Build history of the part. All positions in model axes, mm. A direction names the side the tool comes from. Coordinates: 2 decimals unless noted, no trailing zeros. Loops run counter-clockwise (first coordinate to the right, second up) from the corner with the lowest first, then second, coordinate; pieces in that order, holes last. Notation, with made-up numbers: (47.25, 69) - (56.25, 69) arc R20 ccw to (56.25, 96) - close; hole circle Ø1 at (60.25, 48). An arc over 180 degrees is marked (long way). One line per item, written item: value.
```python
from build123d import *

# Parameters (mm, degrees)
ESBO_O2_R                           = 12.5
RESSALTO_EXTRUS_O1_DEPTH            = 5.55
RESSALTO_EXTRUS_O3_DEPTH            = 3
ESBO_O5_W                           = 25
ESBO_O5_H                           = 7.051040728
RESSALTO_EXTRUS_O4_DEPTH            = 11.8
REBAIXO_PARA_SHCS_M2_51_D           = 2.9
REBAIXO_PARA_SHCS_M2_51_CBORE_D     = 5.5
REBAIXO_PARA_SHCS_M2_51_CBORE_DEPTH = 10
NERVURA1_REACH                      = 67.976
ESBO_O10_WALL_W                     = 145.845066172
ESBO_O10_WALL_H                     = 15
CORTE_EXTRUS_O1_REACH               = 68.009
ESBO_O11_W                          = 9
ESBO_O11_H                          = 8
ESBO_O12_R                          = 3.25
CORTE_EXTRUS_O2_DEPTH               = 67.475439137
ESBO_O13_R                          = 4
CORTE_EXTRUS_O3_DEPTH               = 7.55


with BuildPart() as part:
    # Esboço2 → Ressalto-extrusão1 (new body)
    with BuildSketch(Plane.XY):
        with Locations((-0.474928023, -0.063425095)):
            Circle(ESBO_O2_R)
    extrude(amount=-RESSALTO_EXTRUS_O1_DEPTH)

    # Esboço4 → Ressalto-extrusão3 (add)
    with BuildSketch(Plane(origin=(0, 0, -5.55), x_dir=(-1, 0, 0), z_dir=(0, 0, -1))):
        with BuildLine():
            Line((-12.025071977, -0.063425095), (-12.025071977, 64.120162595))
            Line((-12.025071977, 64.120162595), (12.974928023, 64.120162595))
            Line((12.974928023, 64.120162595), (12.974928023, -0.063425095))
            ThreePointArc((12.974928023, -0.063425095), (0.474928023, -12.563425095), (-12.025071977, -0.063425095))
        make_face()
    extrude(amount=RESSALTO_EXTRUS_O3_DEPTH)

    # Esboço5 → Ressalto-extrusão4 (add)
    with BuildSketch(Plane(origin=(0, 0, -8.55), x_dir=(-1, 0, 0), z_dir=(0, 0, -1))):
        with Locations((0.474928023, 60.594642231)):
            Rectangle(ESBO_O5_W, ESBO_O5_H)
    extrude(amount=-RESSALTO_EXTRUS_O4_DEPTH)

    # Rebaixo para SHCS M2.51 (through all)
    with Locations(Plane(origin=(0, 0, -8.55), x_dir=(-1, 0, 0), z_dir=(0, 0, -1))):
        with Locations((-8.49949915, 61.707782077), (8.5, 61.838275999)):
            CounterBoreHole(REBAIXO_PARA_SHCS_M2_51_D / 2, REBAIXO_PARA_SHCS_M2_51_CBORE_D / 2, REBAIXO_PARA_SHCS_M2_51_CBORE_DEPTH)

    # Esboço10 wall → Nervura1 (add, up to next)
    with BuildSketch(Plane(origin=(0, 53.069121867, -1.15), x_dir=(0, -0.672672793996, -0.739940073396), z_dir=(0, 0.739940073396, -0.672672793996)), mode=Mode.PRIVATE) as nervura1_sk1:
        Rectangle(ESBO_O10_WALL_W, ESBO_O10_WALL_H)
    nervura1_tool1 = extrude(nervura1_sk1.sketch, amount=NERVURA1_REACH, mode=Mode.PRIVATE) - part.part
    add(nervura1_tool1.solids().sort_by_distance((0, 53.069121867, -1.15))[0])

    # Esboço11 → Corte-extrusão1 (cut, up to next)
    with BuildSketch(Plane.XY.offset(-5.55), mode=Mode.PRIVATE) as corte_extrus_o1_sk1:
        with Locations((0, 53.069121867)):
            Rectangle(ESBO_O11_W, ESBO_O11_H)
    corte_extrus_o1_tool1 = extrude(corte_extrus_o1_sk1.sketch, amount=CORTE_EXTRUS_O1_REACH, mode=Mode.PRIVATE) & part.part
    add(corte_extrus_o1_tool1.solids().sort_by_distance((0, 53.069122, -5.55))[0], mode=Mode.SUBTRACT)

    # Esboço12 → Corte-extrusão2 (cut, through all)
    with BuildSketch(Plane(origin=(0, 0, -8.55), x_dir=(-1, 0, 0), z_dir=(0, 0, -1))):
        with Locations((0.474928023, -0.063425095)):
            Circle(ESBO_O12_R)
    extrude(amount=-CORTE_EXTRUS_O2_DEPTH, mode=Mode.SUBTRACT)

    # Esboço13 → Corte-extrusão3 (cut)
    with BuildSketch(Plane(origin=(0, 0, -8.55), x_dir=(-1, 0, 0), z_dir=(0, 0, -1))):
        with Locations((0.474928023, -0.063425095)):
            Circle(ESBO_O13_R)
    extrude(amount=-CORTE_EXTRUS_O3_DEPTH, mode=Mode.SUBTRACT)


solid = part.part
```
Item 1: Cut at C-C, the plane z = -7. Write the cut outline in (x, y), then the cut area to 3 significant figures.
Check result:
outline: (-12.97, -0.06) arc R12.5 ccw to (12.03, -0.06) - (12.03, 64.12) - (9.82, 64.12) arc R2.75 cw (long way) to (7.18, 64.12) - (-6.97, 64.12) arc R2.75 cw (long way) to (-10.03, 64.12) - (-12.97, 64.12) - close; hole circle Ø8 at (-0.47, -0.06)
area: 1,750 mm^2
Item 2: Cut at D-D, the plane y = 50. Write the cut outline in (x, z), then the cut area to 3 significant figures.
Check result:
outline: (-12.97, -8.55) - (12.03, -8.55) - (12.03, -5.55) - (7.5, -5.55) - (7.5, -4.53) - (4.5, -4.53) - (4.5, -5.55) - (-4.5, -5.55) - (-4.5, -4.53) - (-7.5, -4.53) - (-7.5, -5.55) - (-12.97, -5.55) - close
area: 81.1 mm^2
Item 3: Cut at B-B, the plane x = -8.5. Write the cut outline in (y, z), then the cut area to 3 significant figures.
Check result:
outline: (-9.65, -8.55) - (59.09, -8.55) - (59.09, 1.45) - (60.39, 1.45) - (60.39, 3.25) - (57.07, 3.25) - (57.07, -5.55) - (9.52, -5.55) - (9.52, 0) - (-9.65, 0) - close; (63.29, 1.45) - (64.12, 1.45) - (64.12, 3.25) - (63.29, 3.25) - close
area: 334 mm^2
Item 4: Drop flat-ended pins along their axis: P1, Ø3.5, axis at x = 10.5, z = -0.5, coming from the -Y side; P2, Ø4, axis at x = -8.5, y = 61.84, coming from the -Z side; P3, Ø2.5, axis at y = 55, z = -1, coming from the +X side. Give the stop position or say it passes through.
Check result:
P1: stops at y = -8.5
P2: stops at z = 1.45
P3: stops at x = 7.5
Item 5: Tool access for faces 4 (the face through (-2.321, -3.612, -4.828)), 5 (the face through (7.5, 55, -3)), 6 (the face through (2, -3, 0)), 7 (the face through (0, 57.069, -1)): list every direction of +Z, -Z, +X, -X, +Y, -Y with a clear straight run to the whole face (end or side of a thin tool).
Check result:
face 4: -Z
face 5: +Z, +X
face 6: +Z, +X, -X, -Y
face 7: +Z
Item 6: Probe probe 1 along X at (y, z) = (56, -2.75); probe 2 along Y at (x, z) = (-8.5, 2.4); probe 3 along Y at (x, z) = (6, -3). List the from-to ranges inside material, lowest first. Write a range as from..to.
Check result:
probe 1: x = -7.5..-4.5, 4.5..7.5
probe 2: y = 57.07..60.39, 63.29..64.12
probe 3: y = -10.76..10.63, 51.39..60.56, 62.85..64.12
Item 7: Pull direction Y, two halves, no side cores. Call faces 1 (the face through (-7.5, 55, -3)), 2 (the face through (-1, 26, -8.55)), 3 (the face through (0.23, -3.236, -0.507)): released by +Y, released by -Y, zero draft, split by the parting line, or undercut.
Check result:
face 1: undercut
face 2: zero draft
face 3: undercut
Item 8: Cut at A-A, the plane z = -2.75. Write the cut outline in (x, y).
Check result:
outline: circle Ø25 at (-0.47, -0.06); (-12.97, 57.07) - (-7.5, 57.07) - (-7.5, 51.61) - (-4.5, 51.61) - (-4.5, 57.07) - (4.5, 57.07) - (4.5, 51.61) - (7.5, 51.61) - (7.5, 57.07) - (12.03, 57.07) - (12.03, 64.12) - (9.82, 64.12) arc R2.75 cw (long way) to (7.18, 64.12) - (-6.97, 64.12) arc R2.75 cw (long way) to (-10.03, 64.12) - (-12.97, 64.12) - close; hole circle Ø8 at (-0.47, -0.06)
